The model under review builds one solid part; all positions refer to its coordinate system, in mm. Face numbers are marked on the shaded views. A direction names the side the tool comes from. Coordinates: 2 decimals unless noted, no trailing zeros. Loops run counter-clockwise (first coordinate to the right, second up) from the corner with the lowest first, then second, coordinate; pieces in that order, holes last. Notation, with made-up numbers: (72.5, 39) - (131.5, 39) arc R23 cw to (131.5, 54) - close; hole circle Ø3 at (33.5, 9.25). An arc over 180 degrees is marked (long way). Answer in a Markdown table with one row per item. Add a question column.
(1) For P1, Ø3, axis at y = -2, z = -32.5, coming from the +X side; P2, Ø7, axis at x = -9.09, y = -17.14, coming from the +Z side; P3, Ø8, axis at x = -21, z = -17.5, coming from the -Y side; P4, Ø7, axis at x = 0, y = 0, coming from the -Z side, all flat-tipped, find the tip position at first contact; note any pin that passes through.
(2) Mouldability with a two-part tool opening along X and no side actions: class the marked faces 1 and 2 as +X half, -X half, draft (parallel to the pull), parting line (faces both ways), or undercut.
(3) We need section C-C on y = -26. Write out the cut boundary in (x, z), plus the area to 3 significant figures.
(4) We need section D-D on z = -24.5. Write out the cut boundary in (x, y), plus the area to 3 significant figures.
(5) We need section A-A on x = 0. Write out the cut boundary in (y, z).
(6) For line 1 along Y through (x, z) = (0, -11); line 2 along X through (y, z) = (-0.5, -36); line 3 along Z through (x, y) = (22.5, -22.5), list the stretches that pass through material, from the lowest coordinate up.
(7) Machinability: for the marked faces 3 and 4, which of the approach directions +Z, -Z, +X, -X, +Y, -Y give a long, thin tool a straight path to every point of the face, cutting with its end or side? Answer none if there is none.
(8) We need section B-B on x = 7.5. Write out the cut boundary in (y, z).
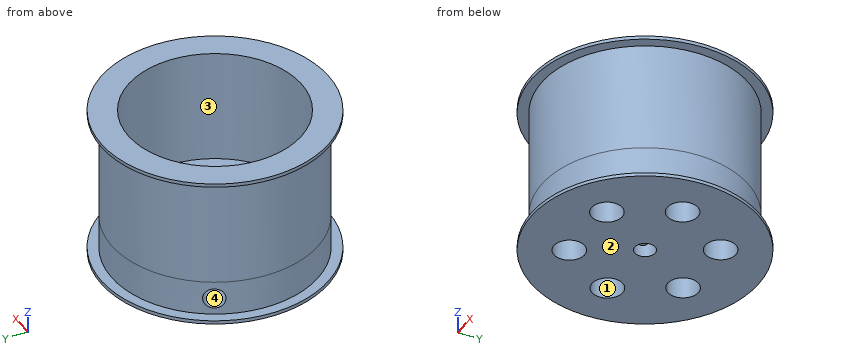
from build123d import *

# Parameters (mm, degrees)
SKETCH1_R           = 32.8
SKETCH1_R_2         = 25
BOSS_EXTRUDE1_DEPTH = 1
BOSS_EXTRUDE2_START = -33
SKETCH2_R           = 29.8
SKETCH2_R_2         = 25
BOSS_EXTRUDE2_DEPTH = 33
BOSS_EXTRUDE3_START = 10
SKETCH3_R           = 29.8
BOSS_EXTRUDE3_DEPTH = 10
BOSS_EXTRUDE4_START = 1
SKETCH4_R           = 32.8
BOSS_EXTRUDE4_DEPTH = 1
SKETCH5_R           = 2.95
CUT_EXTRUDE1_DEPTH  = 64.934966959
SKETCH6_R           = 4.45
CUT_EXTRUDE2_DEPTH  = 64.934966959
SKETCH7_R           = 3
CUT_EXTRUDE3_DEPTH  = 9.4
SKETCH8_R           = 2.5
CUT_EXTRUDE4_DEPTH  = 21


with BuildPart() as part:
    # Sketch1 → Boss-Extrude1 (new body)
    with BuildSketch(Plane.XY):
        Circle(SKETCH1_R)
        Circle(SKETCH1_R_2, mode=Mode.SUBTRACT)
    extrude(amount=BOSS_EXTRUDE1_DEPTH)

    # Sketch2 → Boss-Extrude2 (add)
    with BuildSketch(Plane.XY.offset(1).offset(BOSS_EXTRUDE2_START)):
        Circle(SKETCH2_R)
        Circle(SKETCH2_R_2, mode=Mode.SUBTRACT)
    extrude(amount=BOSS_EXTRUDE2_DEPTH)

    # Sketch3 → Boss-Extrude3 (add)
    with BuildSketch(Plane(origin=(0, 0, -32), x_dir=(-1, 0, 0), z_dir=(0, 0, -1)).offset(BOSS_EXTRUDE3_START)):
        with Locations(Location((0, 0, 0), (0, 0, 180))):
            Circle(SKETCH3_R)
    extrude(amount=-BOSS_EXTRUDE3_DEPTH)

    # Sketch4 → Boss-Extrude4 (add)
    with BuildSketch(Plane(origin=(0, 0, -42), x_dir=(-1, 0, 0), z_dir=(0, 0, -1)).offset(BOSS_EXTRUDE4_START)):
        with Locations(Location((0, 0, 0), (0, 0, 180))):
            Circle(SKETCH4_R)
    extrude(amount=-BOSS_EXTRUDE4_DEPTH)

    # Sketch5 → Cut-Extrude1 (cut, through all)
    with BuildSketch(Plane(origin=(0, 0, -43), x_dir=(-1, 0, 0), z_dir=(0, 0, -1))):
        Circle(SKETCH5_R)
    extrude(amount=-CUT_EXTRUDE1_DEPTH, mode=Mode.SUBTRACT)

    # Sketch6 → Cut-Extrude2 (cut, through all)
    with BuildSketch(Plane(origin=(0, 0, -43), x_dir=(-1, 0, 0), z_dir=(0, 0, -1))):
        with Locations((10.300490658, 16.439583091)):
            Circle(SKETCH6_R)
        with Locations((19.387341913, -0.700695036)):
            Circle(SKETCH6_R)
        with Locations((9.086851255, -17.140278127)):
            Circle(SKETCH6_R)
        with Locations((-10.300490658, -16.439583091)):
            Circle(SKETCH6_R)
        with Locations((-19.387341913, 0.700695036)):
            Circle(SKETCH6_R)
        with Locations((-9.086851255, 17.140278127)):
            Circle(SKETCH6_R)
    extrude(amount=-CUT_EXTRUDE2_DEPTH, mode=Mode.SUBTRACT)

    # Sketch7 → Cut-Extrude3 (cut)
    with BuildSketch(Plane(origin=(-25.807557033, 14.9, 0), x_dir=(0, 0, 1), z_dir=(-0.8660254037844398, 0.499999999999998, 0))):
        with Locations(Location((-37.1, -1.017819827, 0), (0, 0, 270))):
            Circle(SKETCH7_R)
    extrude(amount=-CUT_EXTRUDE3_DEPTH, mode=Mode.SUBTRACT)

    # Sketch8 → Cut-Extrude4 (cut)
    with BuildSketch(Plane(origin=(-17.666918237, 10.2, 0), x_dir=(0, 0, 1), z_dir=(-0.8660254037844398, 0.49999999999999806, 0))):
        with Locations(Location((-37.1, -1.017819827, 0), (0, 0, 270))):
            Circle(SKETCH8_R)
    extrude(amount=-CUT_EXTRUDE4_DEPTH, mode=Mode.SUBTRACT)


solid = part.part
Outcome:
| question | item | result |
|---|---|---|
| 1 | P1 | x = 29.8 |
| 1 | P2 | through |
| 1 | P3 | y = -24.48 |
| 1 | P4 | z = -43 |
| 2 | face 1 | undercut |
| 2 | face 2 | draft |
| 3 | outline | (-20, -43) - (20, -43) - (20, -42) - (14.56, -42) - (14.56, 0) - (20, 0) - (20, 1) - (-20, 1) - (-20, 0) - (-14.56, 0) - (-14.56, -42) - (-20, -42) - close |
| 3 | area | 1,300 mm² |
| 4 | outline | circle Ø59.6 at (0, 0); hole circle Ø50 at (0, 0) |
| 4 | area | 826 mm² |
| 5 | outline | (-32.8, -43) - (-2.95, -43) - (-2.95, -32) - (-25, -32) - (-25, 1) - (-32.8, 1) - (-32.8, 0) - (-29.8, 0) - (-29.8, -42) - (-32.8, -42) - close; (2.95, -43) - (32.8, -43) - (32.8, -42) - (29.8, -42) - (29.8, 0) - (32.8, 0) - (32.8, 1) - (25, 1) - (25, -32) - (2.95, -32) - close |
| 6 | line 1 | -29.8 to -25, 25 to 29.8 |
| 6 | line 2 | -29.8 to -23.83, -14.94 to -5.66, 2.91 to 15.1, 23.67 to 29.8 |
| 6 | line 3 | -43 to -42, 0 to 1 |
| 7 | face 3 | +Z |
| 7 | face 4 | none |
| 8 | outline | (-31.93, -43) - (-19.9, -43) - (-19.9, -32) - (-23.85, -32) - (-23.85, 1) - (-31.93, 1) - (-31.93, 0) - (-28.84, 0) - (-28.84, -42) - (-31.93, -42) - close; (-12.98, -43) - (12.98, -43) - (12.98, -32) - (-12.98, -32) - close; (21.3, -43) - (31.93, -43) - (31.93, -42) - (28.84, -42) - (28.84, 0) - (31.93, 0) - (31.93, 1) - (23.85, 1) - (23.85, -32) - (21.3, -32) - close |
